from build123d import *

# Parameters (mm, degrees)
SKETCH_1_R      = 2
EXTRUDE_1_DEPTH = 5


with BuildPart() as part:
    # 草图1 → 凸台-拉伸1 (new body)
    with BuildSketch(Plane.XY):
        with BuildLine():
            Line((0, 12), (116, 12))
            ThreePointArc((116, 12), (128, 0), (116, -12))
            Line((116, -12), (0, -12))
            ThreePointArc((0, -12), (-12, 0), (0, 12))
        make_face()
        with Locations((49, 0)):
            Circle(SKETCH_1_R, mode=Mode.SUBTRACT)
        Circle(SKETCH_1_R, mode=Mode.SUBTRACT)
        with Locations((10, 0)):
            Circle(SKETCH_1_R, mode=Mode.SUBTRACT)
        with BuildLine():
            Line((23, 4), (39, 4))
            ThreePointArc((39, 4), (43, 0), (39, -4))
            Line((39, -4), (23, -4))
            ThreePointArc((23, -4), (19, 0), (23, 4))
        make_face(mode=Mode.SUBTRACT)
        with BuildLine():
            Line((59, 4), (79, 4))
            ThreePointArc((79, 4), (83, 0), (79, -4))
            Line((79, -4), (59, -4))
            ThreePointArc((59, -4), (55, 0), (59, 4))
        make_face(mode=Mode.SUBTRACT)
        with BuildLine():
            Line((108, 2), (116, 2))
            ThreePointArc((116, 2), (118, 0), (116, -2))
            Line((116, -2), (108, -2))
            ThreePointArc((108, -2), (106, 0), (108, 2))
        make_face(mode=Mode.SUBTRACT)
        with BuildLine():
            Line((88, 2), (96, 2))
            ThreePointArc((96, 2), (98, 0), (96, -2))
            Line((96, -2), (88, -2))
            ThreePointArc((88, -2), (86, 0), (88, 2))
        make_face(mode=Mode.SUBTRACT)
    extrude(amount=EXTRUDE_1_DEPTH)


solid = part.part
Could you check a few things on this model? Use its own coordinates, in mm. A direction names the side the tool comes from. Coordinates: 2 decimals unless noted, no trailing zeros. Order: outer loops, then holes, each group sorted by start corner. A loop starts at its lowest first (then second) coordinate and runs counter-clockwise, first axis right, second up. Notation, with made-up numbers: (-11.5, 1) -> (12.5, 1) arc R10 ccw to (12.5, 12) -> close; hole circle Ø3 at (17, 33.5). An arc over 180 degrees is marked (long way). One line per question, with ' | ' between items.
Q1. Imagine slicing it at C-C on z = 3.1. Please give me the cut outline in (x, y), and give its area (3 significant figures).
Return value:
outline: (0, -12) -> (116, -12) arc R12 ccw to (116, 12) -> (0, 12) arc R12 ccw to start; hole circle Ø4 at (0, 0); hole circle Ø4 at (10, 0); hole (23, -4) -> (39, -4) arc R4 ccw to (39, 4) -> (23, 4) arc R4 ccw to start; hole circle Ø4 at (49, 0); hole (59, -4) -> (79, -4) arc R4 ccw to (79, 4) -> (59, 4) arc R4 ccw to start; hole (88, -2) -> (96, -2) arc R2 ccw to (96, 2) -> (88, 2) arc R2 ccw to start; hole (108, -2) -> (116, -2) arc R2 ccw to (116, 2) -> (108, 2) arc R2 ccw to start | area: 2,720 mm²
Q2. I'm going to push flat-ended pins straight in: P1, Ø3.5, axis at x = 49, y = 0, coming from the -Z side; P2, Ø3, axis at y = -5.5, z = 1.5, coming from the -X side; P3, Ø1.5, axis at y = -7.5, z = 2, coming from the -X side. Where does each tip first touch, or does it pass through?
Return value:
P1: through | P2: x = -11.31 | P3: x = -9.92
Q3. Imagine slicing it at D-D on x = 89.5. Please give me the cut outline in (y, z).
Return value:
outline: (-12, 0) -> (-2, 0) -> (-2, 5) -> (-12, 5) -> close; (2, 0) -> (12, 0) -> (12, 5) -> (2, 5) -> close
Q4. Imagine slicing it at A-A on y = 0. State how many separate pieces and enclosed holes the cut face has, and give its area (3 significant figures).
Return value:
separate pieces: 8 | enclosed holes: 0 | area: 260 mm²
Q5. Thinking about a two-plate mould opening in X: for faces 3 (the face through (59, -5, 0)), 4 (the face through (128, 0, 2)), 5 (the face through (83, 0, 2)), 6 (the face through (55, 0, 2)), which applies, pulls with the +X half, pulls with the -X half, needs draft (parallel to the pull), parting line crosses it, or undercut?
Return value:
face 3: needs draft | face 4: pulls with the +X half | face 5: undercut | face 6: undercut
Q6. If I drill on L1, parallel to Y at x = 10, z = 1.3; L2, parallel to Y at x = 36, z = 2.9; L3, parallel to X at y = -6, z = 4.2, over which ranges is the centre line in solid material (lowest first)?
Return value:
L1: -12 to -2, 2 to 12 | L2: -12 to -4, 4 to 12 | L3: -10.39 to 126.39
Q7. On a 3-axis mill with a long thin cutter (end or side, diameter ignored), from which of +Z, -Z, +X, -X, +Y, -Y can I reach the whole of each face in a straight line? I mean faces 1 (the face through (112, 2, 2)), 2 (the face through (59, -12, 2)). Say none if no direction works.
Return value:
face 1: +Z, -Z | face 2: +Z, -Z, +X, -X, -Y
Q8. Imagine slicing it at B-B on x = 28.5. Please give me the cut outline in (y, z).
Return value:
outline: (-12, 0) -> (-4, 0) -> (-4, 5) -> (-12, 5) -> close; (4, 0) -> (12, 0) -> (12, 5) -> (4, 5) -> close
